```python
from build123d import *

# Parameters (mm, degrees)
F0_W     = 16.8275
F0_H     = 22.170253424
F0_H_2   = 35.886526576
F2_R     = 5.08
F3_R     = 2.54
F4_R     = 2.54
F5_R     = 12.7
F6_DEPTH = 25.4


with BuildPart() as f1:
    # F0 (on Front) → F1 (revolve)
    with BuildSketch(Plane.XZ):
        with Locations((-8.41375, 11.085126712)):
            Rectangle(F0_W, F0_H)
        with Locations((-8.41375, 40.113516712)):
            Rectangle(F0_W, F0_H_2)
        Polygon((-25.4, 22.170253424), (-16.8275, 0), (-16.8275, 22.170253424), align=None)
        Polygon((-25.4, 22.170253424), (-16.8275, 22.170253424), (-16.8275, 58.05678), align=None)
    revolve(axis=Axis((0, 0, 40.113516712), (0, 0, -1)))

    # F2
    f2_edges = [f1.edges().sort_by_distance(p)[0] for p in [
        (25.4, 0, 22.170253),
    ]]
    fillet(f2_edges, radius=F2_R)

    # F3
    f3_edges = [f1.edges().sort_by_distance(p)[0] for p in [
        (-20.828657, 0, 10.347817),
        (24.829814, 0, 20.695635),
        (16.8275, 0, 0),
    ]]
    fillet(f3_edges, radius=F3_R)

    # F4
    f4_edges = [f1.edges().sort_by_distance(p)[0] for p in [
        (16.8275, 0, 58.05678),
    ]]
    fillet(f4_edges, radius=F4_R)

    # F5 (on face) → F6 (cut)
    with BuildSketch(Plane.XY.offset(58.05678)):
        Circle(F5_R)
    extrude(amount=-F6_DEPTH, mode=Mode.SUBTRACT)


solid = f1.part
```
CAD build for the part. Positions are in the model's coordinates, mm. A direction names the side the tool comes from. Coordinates: 2 decimals unless noted, no trailing zeros. Write each loop counter-clockwise with the first axis right and the second up, starting at its lowest first coordinate (ties: lowest second). Pieces come first, ordered by that corner, then holes. Notation, with made-up numbers: (-31.75, 36.5) -> (-13.75, 36.5) arc R18 cw to (-13.75, 49.5) -> close; hole circle Ø11 at (51.5, 82). An arc over 180 degrees is marked (long way). Return JSON: item names as keys, results as strings. Group by question number.
Q1. Flat gauge pins, fed straight in: pin 1 (6 mm diameter, centred on x = -15, z = 31, fed in from +Y); pin 2 (5 mm diameter, centred on y = 1, z = 43.5, fed in from -X); pin 3 (10 mm diameter, centred on y = 18, z = 51, fed in from -X). Where does each tip first touch, or does it go through?
Q2. Pull direction Y, two halves, no side cores. Call faces 3 (the face through (-2.75, -12.4, 45.53)), 4 (the face through (-11, 7, 58.057)), 5 (the face through (-10.94, 17.17, 43.28)): released by +Y, released by -Y, zero draft, split by the parting line, or undercut.
Q3. Which spindle directions (+Z, -Z, +X, -X, +Y, -Y) get a long thin tool onto all of the face, cutting with end or side? Do faces 1 (the face through (0, 0, 0)), 2 (the face through (0, 0, 32.657)). Say none if no direction does.
Q4. Cut at A-A, the plane z = 10. Give the cut face in (x, y), then the cut area to 3 significant figures.
Q5. Cut at B-B, the plane z = 50. Give the cut face in (x, y).
Q6. Drill centre lines: line 1 (Z direction, x = 8, y = -4.5); line 2 (X direction, y = -4, z = 48); line 3 (Y direction, x = 0, z = 38.5). Where is each one in solid material? Low to high.
Returned:
{
 "1": {"pin 1": "stops at y = 20.15", "pin 2": "stops at x = -20.89", "pin 3": "stops at x = -13.46"},
 "2": {"face 3": "undercut", "face 4": "zero draft", "face 5": "split by the parting line"},
 "3": {"face 1": "-Z, +X, -X, +Y, -Y", "face 2": "+Z"},
 "4": {"outline": "circle Ø41.39 at (0, 0)", "area": "1,350 mm2"},
 "5": {"outline": "circle Ø37.5 at (0, 0); hole circle Ø25.4 at (0, 0)"},
 "6": {"line 1": "z = 0 to 32.66", "line 2": "x = -18.81 to -12.05, 12.05 to 18.81", "line 3": "y = -21.5 to -12.7, 12.7 to 21.5"}
}
